Job drawing, mm, ordinate dimensions from the low corner. One solid piece. Round coordinates to 2 decimals unless told otherwise and drop trailing zeros. Write each loop counter-clockwise with the first axis right and the second up, starting at its lowest first coordinate (ties: lowest second). Pieces come first, ordered by that corner, then holes. Notation, with made-up numbers: (76, 32.5) -> (111, 32.5) arc R31 ccw to (111, 59.5) -> close; hole circle Ø6 at (-33.75, 30.5). An arc over 180 degrees is marked (long way). Use CSV: the item, a comma, the result in double quotes. Start each with the question number.
(1) Saw through at B-B (y = 29). Give the cut face in (x, z), plus the area to 3 significant figures.
(2) Drop a flat-ended pin along its axis: pin 1 (1.3 mm diameter, centred on x = 99.5, y = 4.5, fed in from -Z). Give the stop position or say it passes through.
(3) Saw through at D-D (y = 5). Give the cut face in (x, z), plus the area to 3 significant figures.
(4) Saw through at A-A (z = 0.4). Give the cut face in (x, y).
(5) Saw through at C-C (y = 45). Give the cut face in (x, z).
(6) Probe line 1 (X direction, y = 22, z = 1.2); line 2 (Y direction, x = 45, z = 1.9); line 3 (Z direction, x = 100, y = 47). List the from-to ranges inside material, lowest first. Write a range as [from, to].
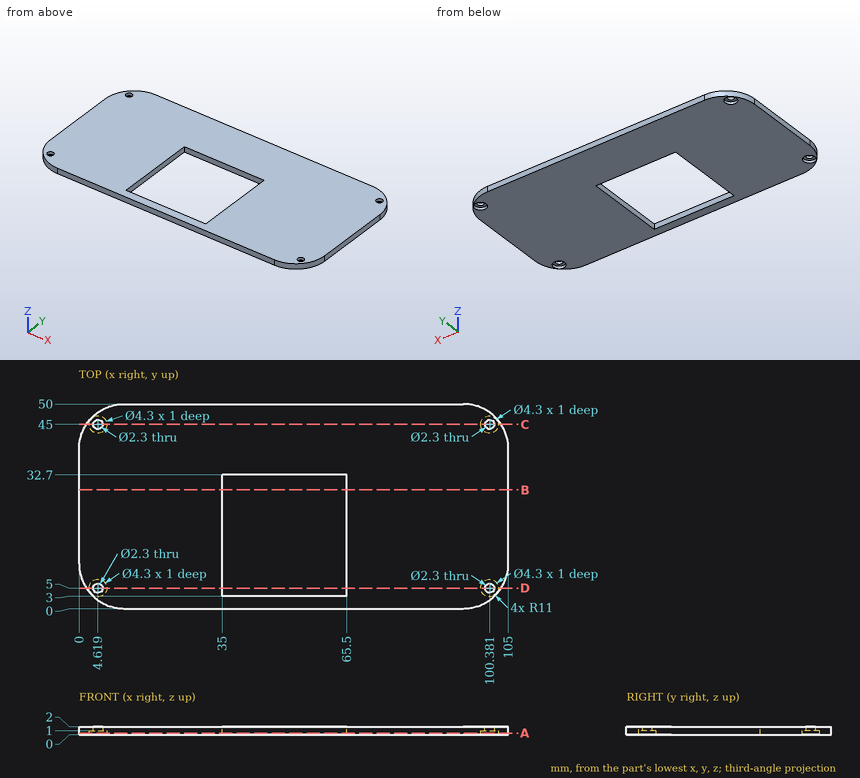
Answers:
1,outline,"(0, 0) -> (35, 0) -> (35, 2) -> (0, 2) -> close; (65.5, 0) -> (105, 0) -> (105, 2) -> (65.5, 2) -> close"
1,area,"149 mm²"
2,pin 1,"stops at z = 1"
3,outline,"(1.78, 0) -> (2.47, 0) -> (2.47, 1) -> (3.47, 1) -> (3.47, 2) -> (1.78, 2) -> close; (5.77, 1) -> (6.77, 1) -> (6.77, 0) -> (35, 0) -> (35, 2) -> (5.77, 2) -> close; (65.5, 0) -> (98.23, 0) -> (98.23, 1) -> (99.23, 1) -> (99.23, 2) -> (65.5, 2) -> close; (101.53, 1) -> (102.53, 1) -> (102.53, 0) -> (103.22, 0) -> (103.22, 2) -> (101.53, 2) -> close"
3,area,"129 mm²"
4,outline,"(0, 11) arc R11 ccw to (11, 0) -> (94, 0) arc R11 ccw to (105, 11) -> (105, 39) arc R11 ccw to (94, 50) -> (11, 50) arc R11 ccw to (0, 39) -> close; hole circle Ø4.3 at (4.62, 5); hole circle Ø4.3 at (4.62, 45); hole (35, 3) -> (65.5, 3) -> (65.5, 32.7) -> (35, 32.7) -> close; hole circle Ø4.3 at (100.38, 5); hole circle Ø4.3 at (100.38, 45)"
5,outline,"(1.78, 0) -> (2.47, 0) -> (2.47, 1) -> (3.47, 1) -> (3.47, 2) -> (1.78, 2) -> close; (5.77, 1) -> (6.77, 1) -> (6.77, 0) -> (98.23, 0) -> (98.23, 1) -> (99.23, 1) -> (99.23, 2) -> (5.77, 2) -> close; (101.53, 1) -> (102.53, 1) -> (102.53, 0) -> (103.22, 0) -> (103.22, 2) -> (101.53, 2) -> close"
6,line 1,"x = [0, 35], [65.5, 105]"
6,line 2,"y = [0, 3], [32.7, 50]"
6,line 3,"z = [1, 2]"
